```python
from build123d import *

# Parameters (mm, degrees)
F4_DEPTH  = 18
F2_R      = 1.75
F2_R_2    = 11.75
F5_DEPTH  = 8
F3_R      = 2
F3_R_2    = 1.75
F3_R_3    = 2.5
F3_R_4    = 11.75
F6_DEPTH  = 3
F7_DEPTH  = 18
F8_R      = 4.5
F8_R_2    = 1.75
F9_DEPTH  = 5
F10_DEPTH = 5
F11_R     = 3.5
F12_DEPTH = 5
F13_DEPTH = 5
F14_DEPTH = 5


with BuildPart() as f4:
    # F1 (on Top) → F4 (new body)
    with BuildSketch(Plane.XY):
        Polygon((-17.59793, 20.648238), (-20.648238, 17.59793), (-20.648238, -17.59793), (-17.59793, -20.648238), (17.59793, -20.648238), (20.648238, -17.59793), (20.648238, 17.59793), (17.59793, 20.648238), align=None)
        Polygon((-15.243323, -17.885499), (-17.885499, -15.243323), (-17.885499, 15.243323), (-15.243323, 17.885499), (15.243323, 17.885499), (17.885499, 15.243323), (17.885499, -15.243323), (15.243323, -17.885499), align=None, mode=Mode.SUBTRACT)
    extrude(amount=F4_DEPTH)

    # F2 (on Top) → F5 (join)
    with BuildSketch(Plane.XY):
        Polygon((-15.243323, 17.885499), (-17.885499, 15.243323), (-17.885499, -15.243323), (-15.243323, -17.885499), (15.243323, -17.885499), (17.885499, -15.243323), (17.885499, 15.243323), (15.243323, 17.885499), align=None)
        with Locations((-13, -13)):
            Circle(F2_R, mode=Mode.SUBTRACT)
        with Locations((13, -13)):
            Circle(F2_R, mode=Mode.SUBTRACT)
        Circle(F2_R_2, mode=Mode.SUBTRACT)
        with Locations((-13, 13)):
            Circle(F2_R, mode=Mode.SUBTRACT)
        with Locations((13, 13)):
            Circle(F2_R, mode=Mode.SUBTRACT)
    extrude(amount=F5_DEPTH)

    # F3 (on Top) → F6 (join)
    with BuildSketch(Plane.XY):
        Polygon((-29.698485, 0), (0, -29.698485), (29.698485, 0), (0, 29.698485), align=None)
        with Locations((0, -21.213203)):
            Circle(F3_R, mode=Mode.SUBTRACT)
        with Locations((-13, -13)):
            Circle(F3_R_2, mode=Mode.SUBTRACT)
        with Locations((13, -13)):
            Circle(F3_R_2, mode=Mode.SUBTRACT)
        with Locations((-21.213203, 0)):
            Circle(F3_R_3, mode=Mode.SUBTRACT)
        Circle(F3_R_4, mode=Mode.SUBTRACT)
        with Locations((-13, 13)):
            Circle(F3_R_2, mode=Mode.SUBTRACT)
        with Locations((0, 21.213203)):
            Circle(F3_R_3, mode=Mode.SUBTRACT)
        with Locations((13, 13)):
            Circle(F3_R_2, mode=Mode.SUBTRACT)
        with Locations((21.213203, 0)):
            Circle(F3_R_3, mode=Mode.SUBTRACT)
    extrude(amount=F6_DEPTH)

    # F3 (on Top) → F7 (cut)
    with BuildSketch(Plane.XY):
        with Locations((21.213203, 0)):
            Circle(F3_R_3)
        with Locations((0, 21.213203)):
            Circle(F3_R_3)
        with Locations((0, -21.213203)):
            Circle(F3_R)
        with Locations((-21.213203, 0)):
            Circle(F3_R_3)
    extrude(amount=F7_DEPTH, mode=Mode.SUBTRACT)

    # F8 (on face) + F2 (on Top) → F9 (cut)
    with BuildSketch(Plane(origin=(0, 0, 0), x_dir=(1, 0, 0), z_dir=(0, 0, -1))):
        with Locations((-13, -13)):
            Circle(F8_R)
        with Locations((-13, -13)):
            Circle(F8_R_2, mode=Mode.SUBTRACT)
    with BuildSketch(Plane.XY):
        with Locations((-13, 13)):
            Circle(F2_R)
    extrude(amount=-F9_DEPTH, mode=Mode.SUBTRACT)

    # F8 (on face) + F2 (on Top) → F10 (cut)
    with BuildSketch(Plane(origin=(0, 0, 0), x_dir=(1, 0, 0), z_dir=(0, 0, -1))):
        with Locations((13, 13)):
            Circle(F8_R)
        with Locations((13, 13)):
            Circle(F8_R_2, mode=Mode.SUBTRACT)
    with BuildSketch(Plane.XY):
        with Locations((13, -13)):
            Circle(F2_R)
    extrude(amount=-F10_DEPTH, mode=Mode.SUBTRACT)

    # F11 (on face) → F12 (cut)
    with BuildSketch(Plane.XY.offset(3)):
        with Locations((0, 21.213203)):
            Circle(F11_R)
        with Locations((0, -21.213203)):
            Circle(F11_R)
        with Locations((21.213203, 0)):
            Circle(F11_R)
        with Locations((-21.213203, 0)):
            Circle(F11_R)
    extrude(amount=F12_DEPTH, mode=Mode.SUBTRACT)

    # F8 (on face) → F13 (cut)
    with BuildSketch(Plane(origin=(0, 0, 0), x_dir=(1, 0, 0), z_dir=(0, 0, -1))):
        with Locations((13, -13)):
            Circle(F8_R)
        with Locations((13, -13)):
            Circle(F8_R_2, mode=Mode.SUBTRACT)
    extrude(amount=-F13_DEPTH, mode=Mode.SUBTRACT)

    # F8 (on face) → F14 (cut)
    with BuildSketch(Plane(origin=(0, 0, 0), x_dir=(1, 0, 0), z_dir=(0, 0, -1))):
        with Locations((-13, 13)):
            Circle(F8_R)
        with Locations((-13, 13)):
            Circle(F8_R_2, mode=Mode.SUBTRACT)
    extrude(amount=-F14_DEPTH, mode=Mode.SUBTRACT)


solid = f4.part
```
The model under review builds one solid part; all positions refer to its coordinate system, in mm. A direction names the side the tool comes from. Round coordinates to 2 decimals unless told otherwise and drop trailing zeros. Loops run counter-clockwise (first coordinate to the right, second up) from the corner with the lowest first, then second, coordinate; pieces in that order, holes last.
1) Wall thickness on line 1 along Y through (x, z) = (-13, 3.1); line 2 along X through (y, z) = (13, 6.15); line 3 along Y through (x, z) = (0, 1.4): over which ranges is each line inside the solid? List them lowest first.
Values follow:
line 1: y = -20.65 to -17.5, -8.5 to 8.5, 17.5 to 20.65
line 2: x = -20.65 to -14.75, -11.25 to 11.25, 14.75 to 20.65
line 3: y = -29.7 to -23.21, -19.21 to -11.75, 11.75 to 18.71, 23.71 to 29.7
2) Consider section D-D on z = 2. Give the number of separate pieces and of enclosed holes in the cut face, then the cut area to 3 significant figures.
Values follow:
separate pieces: 1
enclosed holes: 9
area: 1,250 mm2
3) Consider section B-B on z = 10.75. State the section outline as (x, y) points.
Values follow:
outline: (-20.65, -17.6) - (-17.6, -20.65) - (-1.92, -20.65) arc R2 cw to (1.92, -20.65) - (17.6, -20.65) - (20.65, -17.6) - (20.65, -2.44) arc R2.5 cw to (20.65, 2.44) - (20.65, 17.6) - (17.6, 20.65) - (2.44, 20.65) arc R2.5 cw to (-2.44, 20.65) - (-17.6, 20.65) - (-20.65, 17.6) - (-20.65, 2.44) arc R2.5 cw to (-20.65, -2.44) - close; hole (-17.89, -15.24) - (-15.24, -17.89) - (15.24, -17.89) - (17.89, -15.24) - (17.89, 15.24) - (15.24, 17.89) - (-15.24, 17.89) - (-17.89, 15.24) - close
4) Consider section A-A on x = 13. State the section outline as (y, z) points, then the cut area to 3 significant figures.
Values follow:
outline: (-20.65, 0) - (-17.5, 0) - (-17.5, 5) - (-14.75, 5) - (-14.75, 8) - (-17.89, 8) - (-17.89, 18) - (-20.65, 18) - close; (-11.25, 5) - (-8.5, 5) - (-8.5, 0) - (8.5, 0) - (8.5, 5) - (11.25, 5) - (11.25, 8) - (-11.25, 8) - close; (14.75, 5) - (17.5, 5) - (17.5, 0) - (20.65, 0) - (20.65, 18) - (17.89, 18) - (17.89, 8) - (14.75, 8) - close
area: 275 mm2
5) The part is to be moulded in two halves that separate along Y. For faces 1 (the face through (1.66, -20.1, 1.48)), 2 (the face through (0, 24, 3)), 3 (the face through (-13.228, -11.265, 6.479)), 4 (the face through (-10, 20.648, 9)), say which applies: pulls with the +Y half, pulls with the -Y half, needs draft (parallel to the pull), parting line crosses it, or undercut.
Values follow:
face 1: undercut
face 2: needs draft
face 3: undercut
face 4: pulls with the +Y half
6) Clearance check with flat-ended pins moving along their axes: P1, Ø2, axis at y = -7.5, z = 2.5, coming from the +X side; P2, Ø7, axis at x = 13, y = 13, coming from the +Z side; P3, Ø10, axis at y = -13, z = 14, coming from the -X side. State where each tip first meets the part, or that it passes through.
Values follow:
P1: stops at x = 23.2
P2: stops at z = 8
P3: stops at x = -20.65
7) Tool access review of faces 5 (the face through (-16.55, -16.58, 12.93)), 6 (the face through (0, -19, 8)), 7 (the face through (-24, 0, 3)): name each direction out of +Z, -Z, +X, -X, +Y, -Y from which nothing blocks a thin tool from reaching the whole face with its end or side.
Values follow:
face 5: +Z
face 6: -Y
face 7: -X
